from build123d import *

# Parameters (mm, degrees)
BOSS_EXTRUDE3_DEPTH      = 60
CUT_EXTRUDE1_REACH       = 100.764
SKETCH8_W                = 55
SKETCH8_H                = 60.5
BOSS_EXTRUDE4_DEPTH      = 56
BOSS_EXTRUDE7_REACH      = 100.764
SKETCH13_W               = 20
SKETCH13_H               = 40.707899827
CUT_EXTRUDE7_DEPTH       = 3
CUT_EXTRUDE10_DEPTH      = 99.7643787
CUT_EXTRUDE10_DEPTH_BACK = 99.7643787
SKETCH18_R               = 0.815


with BuildPart() as part:
    # Sketch6 → Boss-Extrude3 (new body)
    with BuildSketch(Plane(origin=(0, 0, 0), x_dir=(0, 0, -1), z_dir=(1, 0, 0))):
        Polygon((0, 0), (65.5, 0), (65.5, -43.17583236), align=None)
    extrude(amount=BOSS_EXTRUDE3_DEPTH)

    # Cut-Extrude1: up to this plane
    cut_extrude1_end = Plane(origin=(60, -43.17583236, -65.5), z_dir=(0, 0.8349267049075845, -0.5503611518195697))
    # Sketch8 → Cut-Extrude1 (cut, up to the surface)
    with BuildSketch(Plane(origin=(0, 0, 0), x_dir=(1, 0, 0), z_dir=(0, 1, 0)), mode=Mode.PRIVATE) as cut_extrude1_sk1:
        with Locations((30, 32.75)):
            Rectangle(SKETCH8_W, SKETCH8_H)
    cut_extrude1_tool1 = split(extrude(cut_extrude1_sk1.sketch, amount=-CUT_EXTRUDE1_REACH, mode=Mode.PRIVATE), bisect_by=cut_extrude1_end, keep=Keep.BOTH, mode=Mode.PRIVATE)
    add(cut_extrude1_tool1.solids().sort_by_distance((30, 0, -32.75))[0], mode=Mode.SUBTRACT)

    # Sketch9 → Boss-Extrude4 (add)
    with BuildSketch(Plane(origin=(2.5, 0, 0), x_dir=(0, 0, -1), z_dir=(1, 0, 0))):
        Polygon((2.5, -1.647932533), (2.5, -0.823966266), (63, -40.707899827), (63, -41.527899827), align=None)
    extrude(amount=BOSS_EXTRUDE4_DEPTH)

    # Boss-Extrude7: up to this plane
    boss_extrude7_end = Plane(origin=(58.5, -0.823966266, -2.5), z_dir=(0, -0.8349015528826996, 0.5503993068618971))
    # Sketch11 → Boss-Extrude7 (add, up to the surface)
    with BuildSketch(Plane(origin=(0, 0, 0), x_dir=(1, 0, 0), z_dir=(0, 1, 0)), mode=Mode.PRIVATE) as boss_extrude7_sk1:
        Polygon((57.5, 63), (57.5, 22.5), (40.834621514, 63), align=None)
    boss_extrude7_tool1 = split(extrude(boss_extrude7_sk1.sketch, amount=-BOSS_EXTRUDE7_REACH, mode=Mode.PRIVATE), bisect_by=boss_extrude7_end, keep=Keep.BOTH, mode=Mode.PRIVATE)
    add(boss_extrude7_tool1.solids().sort_by_distance((51.944874, 0, -49.5))[0])
    # Sketch11 → Boss-Extrude7 (add, up to the surface)
    with BuildSketch(Plane(origin=(0, 0, 0), x_dir=(1, 0, 0), z_dir=(0, 1, 0)), mode=Mode.PRIVATE) as boss_extrude7_sk2:
        Polygon((2.5, 63), (2.5, 2.5), (20.834621514, 63), align=None)
    boss_extrude7_tool2 = split(extrude(boss_extrude7_sk2.sketch, amount=-BOSS_EXTRUDE7_REACH, mode=Mode.PRIVATE), bisect_by=boss_extrude7_end, keep=Keep.BOTH, mode=Mode.PRIVATE)
    add(boss_extrude7_tool2.solids().sort_by_distance((8.611541, 0, -42.833333))[0])

    # Sketch13 → Cut-Extrude7 (cut)
    with BuildSketch(Plane.XY.offset(-63)):
        with Locations((30.834621514, -20.353949914)):
            Rectangle(SKETCH13_W, SKETCH13_H)
    extrude(amount=-CUT_EXTRUDE7_DEPTH, mode=Mode.SUBTRACT)

    # Sketch18 → Cut-Extrude10 (cut, two sides: drawn at the far end of the back side and taken through both)
    with BuildSketch(Plane(origin=(0, 0, 0), x_dir=(1, 0, 0), z_dir=(0, 1, 0)).offset(-CUT_EXTRUDE10_DEPTH_BACK)):
        with Locations((60, 15)):
            Circle(SKETCH18_R)
    extrude(amount=CUT_EXTRUDE10_DEPTH + CUT_EXTRUDE10_DEPTH_BACK, mode=Mode.SUBTRACT)


solid = part.part
Could you check a few things on this model? Use its own coordinates, in mm. A direction names the side the tool comes from. Give positions to 0.01 mm unless a question says otherwise; leave off trailing zeros. Order: outer loops, then holes, each group sorted by start corner. A loop starts at its lowest first (then second) coordinate and runs counter-clockwise, first axis right, second up. Notation, with made-up numbers: (89, 29.25) -> (121, 29.25) arc R17 cw to (121, 51.25) -> close; hole circle Ø2 at (1, -22.5). An arc over 180 degrees is marked (long way). Answer in a Markdown table with one row per item. Add a question column.
Item 1: Imagine slicing it at A-A (x = 38). List the corners of the cut face in (y, z) for me.
Item 2: Imagine slicing it at B-B (z = -32.5). List the corners of the cut face in (x, y) for me.
Item 3: Please list where these lines run through material, in increasing order: probe 1 along X at (y, z) = (-8.5, -46.5); probe 2 along Z at (x, y) = (53, -2.5); probe 3 along Z at (x, y) = (48.5, -12.5).
Item 4: Imagine slicing it at C-C (y = -31). List the corners of the cut face in (x, z) for me.
Item 5: I'm going to push flat-ended pins straight in: P1, Ø1.5, axis at x = 19.5, z = -13, coming from the +Y side; P2, Ø12, axis at y = -34.5, z = -43.5, coming from the +X side; P3, Ø3, axis at x = 30, z = -64, coming from the +Y side; P4, Ø0.9, axis at x = 26.5, y = -0.5, coming from the -Z side. Where does each tip first touch, or does it pass through?
Item 6: For faces 1 (the flat face through (31, -40.708, -64)), 2 (the flat face through (13.576, -15.546, -39.049)), 3 (the flat face through (0, -16, -40)), which set-ups out of +Z, -Z, +X, -X, +Y, -Y let a thin tool reach every point of the face, with its end or its side?
Item 7: We'd pull the mould along X, two halves only. Please class faces 4 (the flat face through (16, -21, -65.5)), 5 (the flat face through (40.835, -21, -64)), 6 (the flat face through (60, -4, -9)): pulls with the +X half, pulls with the -X half, needs draft (parallel to the pull), parting line crosses it, or undercut.
Item 8: Imagine slicing it at D-D (x = 4). List the corners of the cut face in (y, z) for me, and give its area (3 significant figures).
Result:
| question | item | result |
|---|---|---|
| 1 | outline | (-43.18, -65.5) -> (-40.71, -65.5) -> (-40.71, -63) -> (-0.82, -2.5) -> (0, -2.5) -> (0, 0) -> close |
| 2 | outline | (0, -21.42) -> (60, -21.42) -> (60, 0) -> (53.39, 0) -> (53.39, -20.6) -> (11.59, -20.6) -> (11.59, 0) -> (0, 0) -> close |
| 3 | probe 1 | 0 to 15.83, 47.62 to 60 |
| 3 | probe 2 | -65.5 to -33.44, -5.04 to -3.79 |
| 3 | probe 3 | -65.5 to -44.37, -20.21 to -18.96 |
| 4 | outline | (0, -65.5) -> (20.83, -65.5) -> (20.83, -63) -> (16.37, -48.27) -> (46.89, -48.27) -> (40.83, -63) -> (40.83, -65.5) -> (60, -65.5) -> (60, -47.03) -> (0, -47.03) -> close |
| 5 | P1 | y = -7.25 |
| 5 | P2 | x = 60 |
| 5 | P3 | y = -40.38 |
| 5 | P4 | z = -2.69 |
| 6 | face 1 | -Z, +Y |
| 6 | face 2 | +Y |
| 6 | face 3 | +Z, -Z, -X, +Y, -Y |
| 7 | face 4 | needs draft |
| 7 | face 5 | undercut |
| 7 | face 6 | pulls with the +X half |
| 8 | outline | (-43.18, -65.5) -> (0, -65.5) -> (0, -7.45) -> (-4.09, -7.45) -> (-0.82, -2.5) -> (0, -2.5) -> (0, 0) -> close |
| 8 | area | 1,400 mm2 |
